Here's the drawing with two shaded views (mm, measured from the low corner). I have some questions. A direction names the side the tool comes from. Coordinates: 2 decimals unless noted, no trailing zeros. Write each loop counter-clockwise with the first axis right and the second up, starting at its lowest first coordinate (ties: lowest second). Pieces come first, ordered by that corner, then holes.
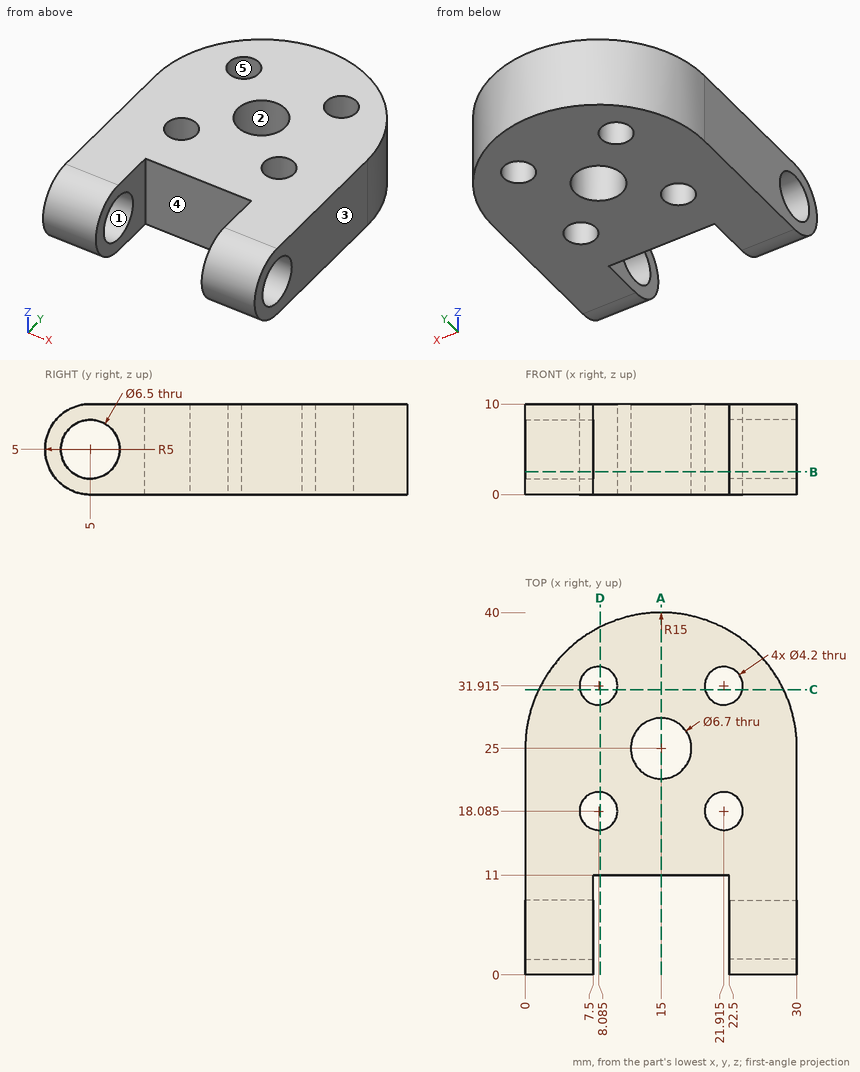
Item 1: Which directions (+Z, -Z, +X, -X, +Y, -Y) give clear straight access to the entire face, cutting with the end or side of a thin tool? Please do the marked faces 4 and 5.
Item 2: I want a section at D-D, the plane x = 8.25. List the corners of the cut face in (y, z) for me.
Item 3: I want a section at C-C, the plane y = 31.5. List the corners of the cut face in (x, z) for me.
Item 4: If we mould it in two halves opening along X, with no side actions, what happens to the marked faces 1, 2 and 3? For each: released by +X, released by -X, zero draft, split by the parting line, or undercut.
Item 5: Will these pins go through, and if not, where does the flat tip stop? pin 1 Ø6 at (y, z) = (5, 5) entering from +X; pin 2 Ø6 at (x, z) = (12, 8.5) entering from +Y; pin 3 Ø6 at (x, z) = (3.5, 6) entering from +Y; pin 4 Ø1.5 at (y, z) = (30.5, 3) entering from -X.
Item 6: If I drill on line 1 along X through (y, z) = (10.5, 1.5); line 2 along X through (y, z) = (18.5, 9); line 3 along X through (y, z) = (22, 8.5), over which ranges is the centre line in solid material (lowest first)?
Item 7: I want a section at A-A, the plane x = 15. List the corners of the cut face in (y, z) for me.
Item 8: I want a section at B-B, the plane z = 2.5. Count the separate pieces of the cut face and the enclosed holes in it.
Taken from the geometry:
1. face 4: +Z, -Z, -Y
1. face 5: +Z, -Z
2. outline: (11, 0) - (15.99, 0) - (15.99, 10) - (11, 10) - close; (20.18, 0) - (29.82, 0) - (29.82, 10) - (20.18, 10) - close; (34.01, 0) - (38.4, 0) - (38.4, 10) - (34.01, 10) - close
3. outline: (1.48, 0) - (6.03, 0) - (6.03, 10) - (1.48, 10) - close; (10.14, 0) - (19.86, 0) - (19.86, 10) - (10.14, 10) - close; (23.97, 0) - (28.52, 0) - (28.52, 10) - (23.97, 10) - close
4. face 1: zero draft
4. face 2: undercut
4. face 3: released by +X
5. pin 1: passes through
5. pin 2: stops at y = 40
5. pin 3: stops at y = 37.36
5. pin 4: stops at x = 0.77
6. line 1: x = 0 to 7.5, 22.5 to 30
6. line 2: x = 0 to 6.03, 10.14 to 19.86, 23.97 to 30
6. line 3: x = 0 to 13.51, 16.49 to 30
7. outline: (11, 0) - (21.65, 0) - (21.65, 10) - (11, 10) - close; (28.35, 0) - (40, 0) - (40, 10) - (28.35, 10) - close
8. separate pieces: 3
8. enclosed holes: 5
